The listing builds one solid part. Answer for the finished solid, in the listing's coordinates (mm). A direction names the side the tool comes from. Coordinates: 2 decimals unless noted, no trailing zeros. Loops run counter-clockwise (first coordinate to the right, second up) from the corner with the lowest first, then second, coordinate; pieces in that order, holes last. Notation, with made-up numbers: (1.25, 74.25) -> (39.25, 74.25) arc R28 ccw to (39.25, 112.25) -> close; hole circle Ø6 at (72.5, 21). An arc over 180 degrees is marked (long way). Answer in a Markdown table with one row per item.
```python
from build123d import *

# Parameters (mm, degrees)
SKETCH1_W            = 31.8
SKETCH1_H            = 13.25
BOSS_EXTRUDE3_DEPTH  = 3
SKETCH3_W            = 31.8
SKETCH3_H            = 3
BOSS_EXTRUDE4_DEPTH  = 24
SKETCH4_W            = 22.8
SKETCH4_H            = 13.25
CUT_EXTRUDE3_DEPTH   = 3
SKETCH6_W            = 31.8
SKETCH6_H            = 2
BOSS_EXTRUDE5_DEPTH  = 13.25
SKETCH7_W            = 3.6
SKETCH7_H            = 3
CUT_EXTRUDE4_DEPTH   = 40.30496947
SKETCH8_W            = 2
SKETCH8_H            = 1.25
BOSS_EXTRUDE6_DEPTH  = 31.8
SKETCH10_W           = 2
SKETCH10_H           = 17.5
CUT_EXTRUDE6_DEPTH   = 38.505207972
BOSS_EXTRUDE7_START  = -31.8
SKETCH11_W           = 3
SKETCH11_H           = 1.25
BOSS_EXTRUDE7_DEPTH  = 31.8
SKETCH12_W           = 22.8
SKETCH12_H           = 1.25
CUT_EXTRUDE7_DEPTH   = 4
SKETCH15_W           = 31.8
SKETCH15_H           = 3
BOSS_EXTRUDE9_DEPTH  = 17.5
BOSS_EXTRUDE12_DEPTH = 5
SKETCH20_W           = 15
SKETCH20_H           = 14.5
SKETCH20_W_2         = 5.230602644
SKETCH20_H_2         = 17.5
CUT_EXTRUDE9_DEPTH   = 100
SKETCH22_R           = 1
SKETCH22_W           = 31.8
SKETCH22_H           = 2.65
CUT_EXTRUDE11_DEPTH  = 20
SKETCH24_R           = 5.925
BOSS_EXTRUDE13_DEPTH = 4.8
SKETCH25_R           = 2.5
BOSS_EXTRUDE14_DEPTH = 2
SKETCH26_W           = 2.9
SKETCH26_H           = 4.9
BOSS_EXTRUDE15_DEPTH = 2.8


with BuildPart() as part:
    # Sketch1 → Boss-Extrude3 (new body)
    with BuildSketch(Plane.XY):
        Rectangle(SKETCH1_W, SKETCH1_H)
    extrude(amount=BOSS_EXTRUDE3_DEPTH)

    # Sketch3 → Boss-Extrude4 (add)
    with BuildSketch(Plane.XY.offset(3)):
        with Locations((0, 8.125)):
            Rectangle(SKETCH3_W, SKETCH3_H)
    extrude(amount=-BOSS_EXTRUDE4_DEPTH)

    # Sketch4 → Cut-Extrude3 (cut)
    with BuildSketch(Plane.XY.offset(3)):
        Rectangle(SKETCH4_W, SKETCH4_H)
    extrude(amount=-CUT_EXTRUDE3_DEPTH, mode=Mode.SUBTRACT)

    # Sketch6 → Boss-Extrude5 (add)
    with BuildSketch(Plane.XZ.offset(-6.625)):
        with Locations((0, -16.4)):
            Rectangle(SKETCH6_W, SKETCH6_H)
    extrude(amount=BOSS_EXTRUDE5_DEPTH)

    # Sketch7 → Cut-Extrude4 (cut, through all)
    with BuildSketch(Plane.ZY.offset(15.9)):
        with Locations((-19.2, 8.125)):
            Rectangle(SKETCH7_W, SKETCH7_H)
    extrude(amount=-CUT_EXTRUDE4_DEPTH, mode=Mode.SUBTRACT)

    # Sketch8 → Boss-Extrude6 (add)
    with BuildSketch(Plane(origin=(15.9, 0, 0), x_dir=(0, 0, -1), z_dir=(1, 0, 0))):
        with Locations((16.4, -7.25)):
            Rectangle(SKETCH8_W, SKETCH8_H)
    extrude(amount=-BOSS_EXTRUDE6_DEPTH)

    # Sketch10 → Cut-Extrude6 (cut, through all)
    with BuildSketch(Plane(origin=(15.9, 0, 0), x_dir=(0, 0, -1), z_dir=(1, 0, 0))):
        with Locations((16.4, 0.875)):
            Rectangle(SKETCH10_W, SKETCH10_H)
    extrude(amount=-CUT_EXTRUDE6_DEPTH, mode=Mode.SUBTRACT)

    # Sketch11 → Boss-Extrude7 (add)
    with BuildSketch(Plane(origin=(15.9, 0, 0), x_dir=(0, 0, -1), z_dir=(1, 0, 0)).offset(BOSS_EXTRUDE7_START)):
        with Locations((-1.5, -7.25)):
            Rectangle(SKETCH11_W, SKETCH11_H)
    boss_extrude7 = extrude(amount=BOSS_EXTRUDE7_DEPTH)

    # Mirror2: Boss-Extrude7 across plane
    add(boss_extrude7.mirror(Plane(origin=(0, 0, 0), x_dir=(0, 0, 1), z_dir=(1, 0, 0))))

    # Sketch12 → Cut-Extrude7 (cut)
    with BuildSketch(Plane.XY.offset(3)):
        with Locations((0, -7.25)):
            Rectangle(SKETCH12_W, SKETCH12_H)
    extrude(amount=-CUT_EXTRUDE7_DEPTH, mode=Mode.SUBTRACT)

    # Sketch15 → Boss-Extrude9 (add)
    with BuildSketch(Plane(origin=(0, 9.625, 0), x_dir=(1, 0, 0), z_dir=(0, 1, 0))):
        with Locations((0, 16.9)):
            Rectangle(SKETCH15_W, SKETCH15_H)
    extrude(amount=-BOSS_EXTRUDE9_DEPTH)

    # Sketch19 → Boss-Extrude12 (add)
    with BuildSketch(Plane.XY.offset(3)):
        Polygon((-15.9, 9.625), (15.9, 9.625), (15.9, -7.875), (11.4, -7.875), (11.4, 6.625), (-11.4, 6.625), (-11.4, -7.875), (-15.9, -7.875), align=None)
    extrude(amount=-BOSS_EXTRUDE12_DEPTH)

    # Sketch20 → Cut-Extrude9 (cut)
    with BuildSketch(Plane.ZY.offset(15.9)):
        with Locations((-7.9, -0.625)):
            Rectangle(SKETCH20_W, SKETCH20_H)
        with Locations((4.215301322, 0.875)):
            Rectangle(SKETCH20_W_2, SKETCH20_H_2)
    extrude(amount=-CUT_EXTRUDE9_DEPTH, mode=Mode.SUBTRACT)

    # Sketch22 → Cut-Extrude11 (cut)
    with BuildSketch(Plane.XY.offset(1.6)):
        with Locations((-14, 0.575)):
            Circle(SKETCH22_R)
        with Locations((14, 0.575)):
            Circle(SKETCH22_R)
        with Locations((0, -6.55)):
            Rectangle(SKETCH22_W, SKETCH22_H)
    extrude(amount=-CUT_EXTRUDE11_DEPTH, mode=Mode.SUBTRACT)

    # Sketch24 → Boss-Extrude13 (add)
    with BuildSketch(Plane(origin=(0, 0, -18.4), x_dir=(-1, 0, 0), z_dir=(0, 0, -1))):
        with Locations(Location((5.47, 0.7, 0), (0, 0, 270))):
            Circle(SKETCH24_R)
    extrude(amount=BOSS_EXTRUDE13_DEPTH)

    # Sketch25 → Boss-Extrude14 (add)
    with BuildSketch(Plane(origin=(0, 0, -23.2), x_dir=(-1, 0, 0), z_dir=(0, 0, -1))):
        with Locations((5.47, 0.7)):
            Circle(SKETCH25_R)
    extrude(amount=BOSS_EXTRUDE14_DEPTH)

    # Sketch26 → Boss-Extrude15 (add)
    with BuildSketch(Plane(origin=(0, 9.625, 0), x_dir=(1, 0, 0), z_dir=(0, 1, 0))):
        with Locations((-8.45, 7.97)):
            Rectangle(SKETCH26_W, SKETCH26_H)
        with Locations((2.6, 7.97)):
            Rectangle(SKETCH26_W, SKETCH26_H)
    extrude(amount=BOSS_EXTRUDE15_DEPTH)


solid = part.part
```
Item 1: Determine the mould class of faces 1 (the face through (0, 1, -15.4)), 2 (the face through (-11.345, 1.471, -20.766)), 3 (the face through (-13.046, 0.875, 0.614)) for opening direction X: +X half, -X half, draft (parallel to the pull), parting line (faces both ways), or undercut.
Findings below:
| item | result |
|---|---|
| face 1 | draft |
| face 2 | parting line |
| face 3 | undercut |
Item 2: A cutting plane is placed at B-B, the plane y = 6.25. Determine the outline of the cut face in (x, z), plus the area to 3 significant figures.
Findings below:
| item | result |
|---|---|
| outline | (-15.9, -18.4) -> (-7.54, -18.4) -> (-7.54, -23.2) -> (-3.4, -23.2) -> (-3.4, -18.4) -> (15.9, -18.4) -> (15.9, -15.4) -> (-15.9, -15.4) -> close; (-15.9, -0.4) -> (-11.4, -0.4) -> (-11.4, 1.6) -> (-15.9, 1.6) -> close; (11.4, -0.4) -> (15.9, -0.4) -> (15.9, 1.6) -> (11.4, 1.6) -> close |
| area | 133 mm2 |
Item 3: Flat-ended cylindrical pins translate along their axes: pin 1 Ø3.5 at (x, y) = (-13.5, 3.5) entering from -Z; pin 2 Ø2 at (x, y) = (3, 11.5) entering from -Z; pin 3 Ø3 at (x, y) = (-8, 11.5) entering from +Z; pin 4 Ø1.8 at (x, y) = (-14, 0.575) entering from -Z. Find the tip coordinate at first contact, or state that the pin passes through.
Findings below:
| item | result |
|---|---|
| pin 1 | stops at z = -18.4 |
| pin 2 | stops at z = -10.42 |
| pin 3 | stops at z = -5.52 |
| pin 4 | passes through |
Item 4: A tool of negligible diameter and unlimited length cuts with its end or side. For faces 4 (the face through (1.15, 11, -8)), 5 (the face through (-6, -2, -23.2)), 6 (the face through (-8, 11, -5.52)), 7 (the face through (11.4, 1, 1)), 8 (the face through (-8, 11, -10.42)), from which of +Z, -Z, +X, -X, +Y, -Y can it reach the whole face along a straight path? Write none if from no direction.
Findings below:
| item | result |
|---|---|
| face 4 | +Z, -Z, +Y |
| face 5 | -Z |
| face 6 | +Z, +X, -X, +Y |
| face 7 | +Z, -Y |
| face 8 | -Z, +X, -X, +Y |
Item 5: Find the intervals of material crossed by probe 1 along Y at (x, z) = (-14, -15.75) (3 decimals); probe 2 along Z at (x, y) = (14.5, -2); probe 3 along X at (y, z) = (-0.25, -17.25), in increasing order.
Findings below:
| item | result |
|---|---|
| probe 1 | y = -5.225 to -0.425, 1.575 to 9.625 |
| probe 2 | z = -18.4 to -15.4, -0.4 to 1.6 |
| probe 3 | x = -15.9 to -14.57, -13.43 to 13.43, 14.57 to 15.9 |
Item 6: A cutting plane is placed at D-D, the plane y = 2.25. Determine the outline of the cut face in (x, z), plus the area to 3 significant figures.
Findings below:
| item | result |
|---|---|
| outline | (-15.9, -18.4) -> (-11.19, -18.4) -> (-11.19, -23.2) -> (-7.43, -23.2) -> (-7.43, -25.2) -> (-3.51, -25.2) -> (-3.51, -23.2) -> (0.25, -23.2) -> (0.25, -18.4) -> (15.9, -18.4) -> (15.9, -15.4) -> (-15.9, -15.4) -> close; (-15.9, -0.4) -> (-11.4, -0.4) -> (-11.4, 1.6) -> (-15.9, 1.6) -> close; (11.4, -0.4) -> (15.9, -0.4) -> (15.9, 1.6) -> (11.4, 1.6) -> close |
| area | 176 mm2 |
Item 7: A cutting plane is placed at C-C, the plane x = 3.5. Determine the outline of the cut face in (y, z) (3 decimals).
Findings below:
| item | result |
|---|---|
| outline | (-5.225, -18.4) -> (9.625, -18.4) -> (9.625, -10.42) -> (12.425, -10.42) -> (12.425, -5.52) -> (9.625, -5.52) -> (9.625, 1.6) -> (6.625, 1.6) -> (6.625, -15.4) -> (-5.225, -15.4) -> close |
Item 8: A cutting plane is placed at A-A, the plane x = 14. Determine the outline of the cut face in (y, z) (3 decimals), plus the area to 3 significant figures.
Findings below:
| item | result |
|---|---|
| outline | (-5.225, -18.4) -> (-0.425, -18.4) -> (-0.425, -15.4) -> (-5.225, -15.4) -> close; (-5.225, -0.4) -> (-0.425, -0.4) -> (-0.425, 1.6) -> (-5.225, 1.6) -> close; (1.575, -18.4) -> (9.625, -18.4) -> (9.625, 1.6) -> (1.575, 1.6) -> (1.575, -0.4) -> (6.625, -0.4) -> (6.625, -15.4) -> (1.575, -15.4) -> close |
| area | 109 mm2 |
